Verification items for the finished model (mm, model axes). A direction names the side the tool comes from. Give positions to 0.01 mm unless a question says otherwise; leave off trailing zeros. Write each loop counter-clockwise with the first axis right and the second up, starting at its lowest first coordinate (ties: lowest second). Pieces come first, ordered by that corner, then holes. Notation, with made-up numbers: (27, -2) - (61, -2) arc R18 ccw to (61, 2) - close; hole circle Ø9 at (-2, 50). An arc over 180 degrees is marked (long way). Answer as a JSON object with one key per item and string values. Group by question number.
Item 1: Scan lines: line 1 along Y through (x, z) = (-14, -1); line 2 along Z through (x, y) = (-27, 10); line 3 along Z through (x, y) = (-72, 9.25). Record each from-to range of solid material in increasing order. Write a range as [from, to].
Item 2: Sectioned sample at C-C, the plane z = -18. Record the boundary of the cut face in (x, y).
Item 3: Go/stop test with flat-tipped pins: pin 1 (6.5 mm diameter, centred on x = -14, y = 7.5, fed in from -Z); pin 2 (7.5 mm diameter, centred on x = -39.5, y = 4.5, fed in from -Z); pin 3 (1 mm diameter, centred on y = 2, z = -19.5, fed in from +X); pin 4 (8 mm diameter, centred on x = -36, z = -9, fed in from -Y). Record where each tip stops, or that it passes through.
Item 4: Draft check along Z on faces 4 (the face through (-80, 7, -21)), 5 (the face through (-54, 0, -14)), 6 (the face through (-67.23, 7.6, -12.47)). Enter one of: +Z half, -Z half, draft (parallel to the pull), parting line (faces both ways), or undercut.
Item 5: Sectioned sample at B-B, the plane y = 7.5. Count the separate pieces of the cut face and the enclosed holes in it, and give its area (3 significant figures).
Item 6: Sectioned sample at A-A, the plane x = -14. Record the boundary of the cut face in (y, z), and give its area (3 significant figures).
Item 7: Tool access check on faces 1 (the face through (-18, 7, -6)), 2 (the face through (-44, 8, -3)), 3 (the face through (-89.566, 5.06, -34.868)). Record the directions out of +Z, -Z, +X, -X, +Y, -Y that give a thin tool (end or side, any length) a straight path to the whole face; none if there is none.
```python
from build123d import *

# Parameters (mm, degrees)
BOSS_EXTRUDE1_DEPTH = 15
FILLET1_R           = 6
CUT_EXTRUDE1_DEPTH  = 111.72308217
SKETCH3_R           = 2.75
CUT_EXTRUDE2_DEPTH  = 109.507513635
SKETCH4_R           = 2.75
CUT_EXTRUDE3_DEPTH  = 104.169159776


with BuildPart() as part:
    # Sketch1 → Boss-Extrude1 (new body)
    with BuildSketch(Plane(origin=(0, 0, 0), x_dir=(1, 0, 0), z_dir=(0, 1, 0))):
        Polygon((0, 0), (-59, 0), (-100.71930009, 41.71930009), (-96.476659403, 45.961940777), (-75.263455967, 24.748737342), (-30, 6), (0, 6), align=None)
    extrude(amount=BOSS_EXTRUDE1_DEPTH)

    # Fillet1
    fillet1_edges = [part.edges().sort_by_distance(p)[0] for p in [
        (-96.476659403, 7.5, -45.961940777),
        (0, 7.5, -6),
    ]]
    fillet(fillet1_edges, radius=FILLET1_R - 0.0001)  # a hair under: the kernel refuses the full size

    # Sketch2 → Cut-Extrude1 (cut, through all)
    with BuildSketch(Plane(origin=(0, 15, 0), x_dir=(1, 0, 0), z_dir=(0, 1, 0))):
        Polygon((-76.962819459, 22.205460146), (-30.596737102, 3), (-57.757359313, 3), align=None)
    extrude(amount=-CUT_EXTRUDE1_DEPTH, mode=Mode.SUBTRACT)

    # Sketch3 → Cut-Extrude2 (cut, through all)
    with BuildSketch(Plane(origin=(0, 0, -6), x_dir=(-1, 0, 0), z_dir=(0, 0, -1))):
        with Locations((14, 7.5)):
            Circle(SKETCH3_R)
    extrude(amount=-CUT_EXTRUDE2_DEPTH, mode=Mode.SUBTRACT)

    # Sketch4 → Cut-Extrude3 (cut, through all)
    with BuildSketch(Plane(origin=(-25.257359313, 0, 25.257359313), x_dir=(-0.7071067811865465, 0, -0.7071067811865487), z_dir=(0.7071067811865487, 0, -0.7071067811865465))):
        with Locations((86.71930009, 7.5)):
            Circle(SKETCH4_R)
    extrude(amount=-CUT_EXTRUDE3_DEPTH, mode=Mode.SUBTRACT)


solid = part.part
```
Geometry check:
{
 "1": {"line 1": "[0, 4.75], [10.25, 15]", "line 2": "[-6, 0]", "line 3": "[-23.4, -20.15], [-17.24, -13]"},
 "2": {"outline": "(-77, 0) - (-72.76, 0) - (-72.76, 15) - (-77, 15) - close; (-66.81, 0) - (-58.97, 0) - (-58.97, 15) - (-66.81, 15) - close"},
 "3": {"pin 1": "z = -6", "pin 2": "z = -11.49", "pin 3": "x = -61.38", "pin 4": "y = 0"},
 "4": {"face 4": "+Z half", "face 5": "draft", "face 6": "undercut"},
 "5": {"separate pieces": "3", "enclosed holes": "1", "area": "599 mm^2"},
 "6": {"outline": "(0, -6) - (4.75, -6) - (4.75, 0) - (0, 0) - close; (10.25, -6) - (15, -6) - (15, 0) - (10.25, 0) - close", "area": "57.0 mm^2"},
 "7": {"face 1": "-Z, +X, +Y, -Y", "face 2": "+Y, -Y", "face 3": "none"}
}
